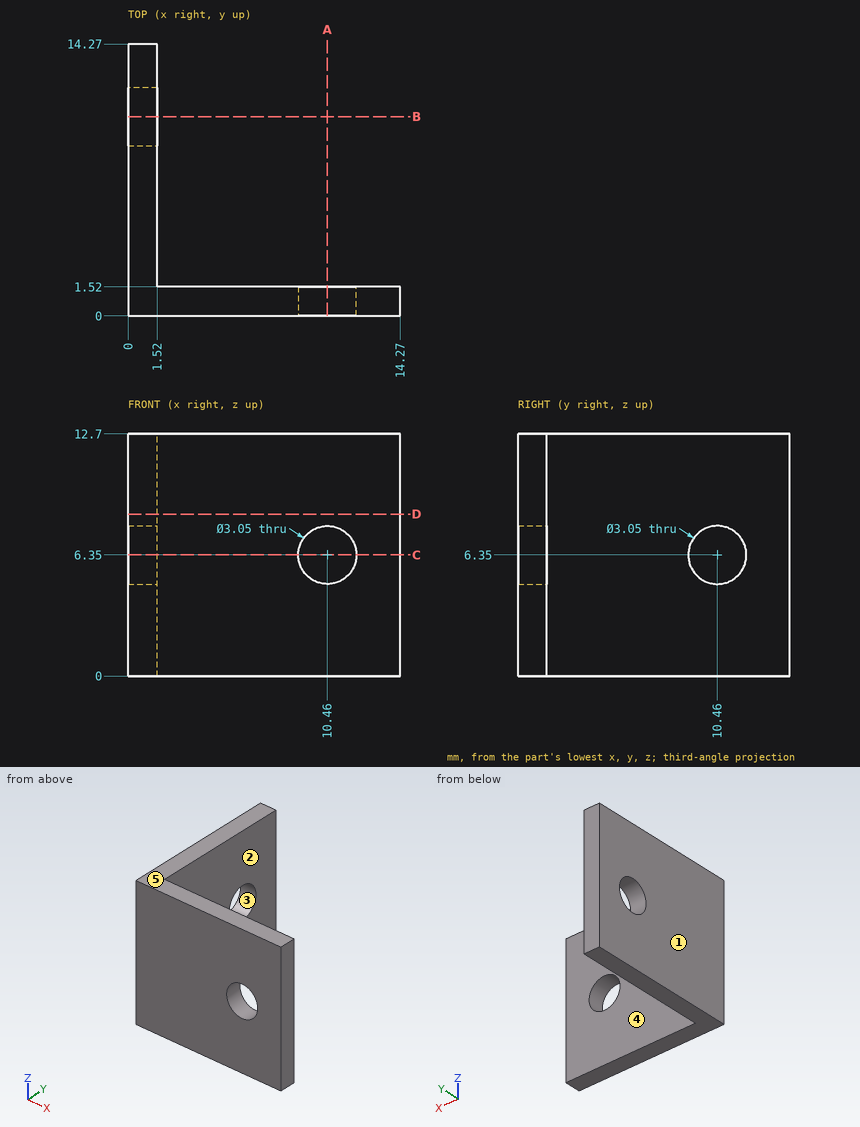
Could you check a few things on this drawing? It's one solid part, dimensions in mm from its lowest x, y, z. A direction names the side the tool comes from. Round coordinates to 2 decimals unless told otherwise and drop trailing zeros. Order: outer loops, then holes, each group sorted by start corner. A loop starts at its lowest first (then second) coordinate and runs counter-clockwise, first axis right, second up.
Q1. Thinking about a two-plate mould opening in Y: for the marked faces 3, 4 and 5, which applies, released by +Y, released by -Y, zero draft, split by the parting line, or undercut?
Geometry says:
face 3: undercut
face 4: released by +Y
face 5: zero draft
Q2. Imagine slicing it at A-A, the plane x = 10.46. List the corners of the cut face in (y, z) for me (3 decimals).
Geometry says:
outline: (0, 0) - (1.52, 0) - (1.52, 4.825) - (0, 4.825) - close; (0, 7.875) - (1.52, 7.875) - (1.52, 12.7) - (0, 12.7) - close
Q3. Which directions (+Z, -Z, +X, -X, +Y, -Y) give clear straight access to the entire face, cutting with the end or side of a thin tool? Please do the marked faces 1 and 2.
Geometry says:
face 1: +Z, -Z, -X, +Y, -Y
face 2: +Z, -Z, +X, +Y
Q4. Imagine slicing it at D-D, the plane z = 8.5. List the corners of the cut face in (x, y) for me.
Geometry says:
outline: (0, 0) - (14.27, 0) - (14.27, 1.52) - (1.52, 1.52) - (1.52, 14.27) - (0, 14.27) - close
Q5. Please list where these lines run through material, in increasing order: probe 1 along Z at (x, y) = (10.46, 0.85) (3 decimals); probe 2 along X at (y, z) = (3, 5.25).
Geometry says:
probe 1: z = 0 to 4.825, 7.875 to 12.7
probe 2: x = 0 to 1.52
Q6. I'm going to push flat-ended pins straight in: P1, Ø4, axis at y = 5.5, z = 4.5, coming from the +X side; P2, Ø3, axis at x = 6.5, z = 3, coming from the +Y side. Where does each tip first touch, or does it pass through?
Geometry says:
P1: stops at x = 1.52
P2: stops at y = 1.52
Q7. Imagine slicing it at C-C, the plane z = 6.35. List the corners of the cut face in (x, y) for me (3 decimals).
Geometry says:
outline: (0, 0) - (8.935, 0) - (8.935, 1.52) - (1.52, 1.52) - (1.52, 8.935) - (0, 8.935) - close; (0, 11.985) - (1.52, 11.985) - (1.52, 14.27) - (0, 14.27) - close; (11.985, 0) - (14.27, 0) - (14.27, 1.52) - (11.985, 1.52) - close
